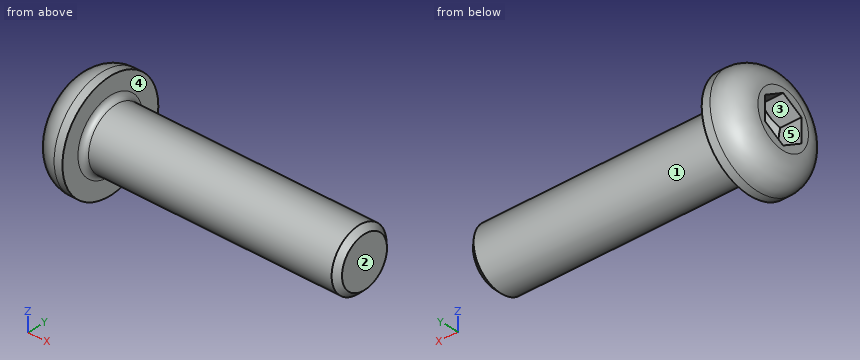
Autodesk Inventor part; units mm, degrees
ref_plane "Work Plane1" through (29, 0, 0) normal (0, -1, 0) x (1, 0, 0)
ref_plane "YZ Plane" through (0, 0, 0) normal (1, 0, 0) x (0, 1, 0)
ref_plane "XZ Plane" through (0, 0, 0) normal (0, 1, 0) x (-1, 0, 0)
sketch "Skizze1" plane through (0, 0, 0) normal (0, 0, 1) x (1, 0, 0)
  line L0 (0.2267, 0) -> (50, 0)
  line L1 (50, 0) -> (50, 6)
  line L2 (50, 6) -> (5.25, 6)
  line L3 (5.25, 6) -> (4.1764, 6)
  line L4 (4.1764, 6) -> (0, 6)
  line L5 (0, 6) -> (0, 10.5)
  line L6 (0, 10.5) -> (-6.6, 10.5)
  line L7 (-6.6, 10.5) -> (-6.6, 4.6188)
  line L8 (-6.6, 4.6188) -> (-2.44, 4.6188)
  line L9 (-2.44, 4.6188) -> (0.2267, 0)
  line L10 (-17.92, 0) -> (61.32, 0)
  line L11 (0, -2.1) -> (0, 12.6)
  line L12 (5.25, 6) -> (0, 6) construction
  dimension "d1" = 44.75
  dimension "d2" = 1.0736
  dimension "d3" = 6.6
  dimension "d4" = 4.16
  dimension "d5" = 60
  dimension "d6" = 12
  dimension "d7" = 12
  dimension "d8" = 9.2376
  dimension "d9" = 21
  dimension "d26" = 50
revolve "Körper" add sketch "Skizze1" angle 360 about axis through (0.2267, 0, 0) along (1, 0, 0) contours L9 L11 L4 L3 L2 L1 L0 | L9 L8 L7 L6 L5 L11
sketch "Skizze2" plane through (-6.6, 0, 0) normal (-1, 0, 0) x (0, 0, 1)
  circle A0 centre (0, 0) radius 4.6188
  line L0 (0, -14.7) -> (0, 14.7)
  line L1 (-14.7, 0) -> (14.7, 0)
  line L2 (4.6188, 0) -> (2.3094, -4)
  line L3 (2.3094, -4) -> (-2.3094, -4)
  line L4 (-2.3094, -4) -> (-4.6188, 0)
  line L5 (-4.6188, 0) -> (-2.3094, 4)
  line L6 (-2.3094, 4) -> (2.3094, 4)
  line L7 (2.3094, 4) -> (4.6188, 0)
extrude "Loch" add sketch "Skizze2" against normal up to next contours L7 A0 | A0 L2 | L6 L0 A0 | A0 L0 L3 | L0 L6 A0 | A0 L3 L0 | L4 A0 | A0 L5
fillet "Rundung1" radius 4.97 1 edges at (-6.6, -10.5, 0)
thread "Gewinde"
chamfer "Fase1" distance 1.0735 distance2 1.0735 1 edges at (50, -6, 0) measured on face at (50, 1.5551, -0.8476)
ref_plane "Work Plane1" through (29, 0, 0) normal (0, -1, 0) x (1, 0, 0)
fillet "Rundung2" radius 1.1 1 edges at (0, -6, 0)
equation "\"d1\" = GEL"
equation "\"d3\" = KOH"
equation "\"d4\" = INTI"
equation "\"d6\" = GD"
equation "\"d7\" = BDM"
equation "\"d8\" = 1.1547 * SW"
equation "\"d9\" = KOD"
equation "\"d26\" = NLG"
equation "\"d17\" = RR"
equation "\"d13\" = GEL"
equation "\"d15\" = -0.5 * SPD + 0.5 * GD"
equation "\"d16\" = GUL"
equation "\"d30\" = R"
equation "\"GD\" = NND"
equation "\"NLG\" = 50"
equation "\"GEL\" = 44.75"
equation "\"KOD\" = 21"
equation "\"KOH\" = 6.6"
equation "\"INTI\" = 4.16"
equation "\"GAL\" = 0.61345 * PTC"
equation "\"GUL\" = 0.61345 * PTC"
equation "\"BDM\" = NND"
equation "\"SW\" = 8"
equation "\"RR\" = 4.97"
equation "\"SPD\" = NND - 1.2269 * PTC"
equation "\"R\" = 1.1"
equation "\"TOA\" = 30deg"
equation "\"GD1\" = THREADDIA - 1.2269 * PTC"
equation "\"THREADDIA\" = 12"
equation "\"PTC\" = 1.75"
equation "\"NND\" = 12"
equation "\"KOH1\" = 1.63"
equation "\"E0\" = 9.149"
properties part number "ISO 7380-1 - M12 x 50" material "Stahl"
Design review of the part built by this model. Coordinates are the model's own, in mm. Face numbers are marked on the shaded views. A direction names the side the tool comes from. Coordinates: 2 decimals unless noted, no trailing zeros. Loops run counter-clockwise (first coordinate to the right, second up) from the corner with the lowest first, then second, coordinate; pieces in that order, holes last. Notation, with made-up numbers: (25.5, 57.5) - (84.5, 57.5) arc R20 ccw to (84.5, 95.5) - close; hole circle Ø4 at (50.25, -6.5). An arc over 180 degrees is marked (long way). Use CSV: the item, a comma, the result in double quotes. Start each with the question number.
1) Tool access review of the marked faces 4 and 5: name each direction out of +Z, -Z, +X, -X, +Y, -Y from which nothing blocks a thin tool from reaching the whole face with its end or side.
2) Wall thickness on L1, parallel to Y at x = 35, z = 0.25; L2, parallel to X at y = 7, z = 7; L3, parallel to Z at x = 20, y = -5.25: over which ranges is each line inside the solid? List them lowest first. Write a range as from..to.
3) The part is to be moulded in two halves that separate along Y. For the marked faces 1, 2 and 3, say which applies: +Y half, -Y half, draft (parallel to the pull), parting line (faces both ways), or undercut.
4) For pin 1 Ø8 at (x, z) = (35, -5.5) entering from +Y; pin 2 Ø2 at (y, z) = (2, 6) entering from -X; pin 3 Ø12 at (x, y) = (30, 4.5) entering from -Z; pin 4 Ø6 at (x, z) = (10, -2.5) entering from -Y, all flat-tipped, find the tip position at first contact; note any pin that passes through.
5) Consider section A-A on x = 29. Write out the cut boundary in (y, z).
Geometry says:
1,face 4,"+X"
1,face 5,"-X"
2,L1,"-5.99..5.99"
2,L2,"-4..0"
2,L3,"-2.9..2.9"
3,face 1,"parting line"
3,face 2,"draft"
3,face 3,"undercut"
4,pin 1,"y = 5.81"
4,pin 2,"x = -6.6"
4,pin 3,"z = -6"
4,pin 4,"y = -6"
5,outline,"circle Ø12 at (0, 0)"
